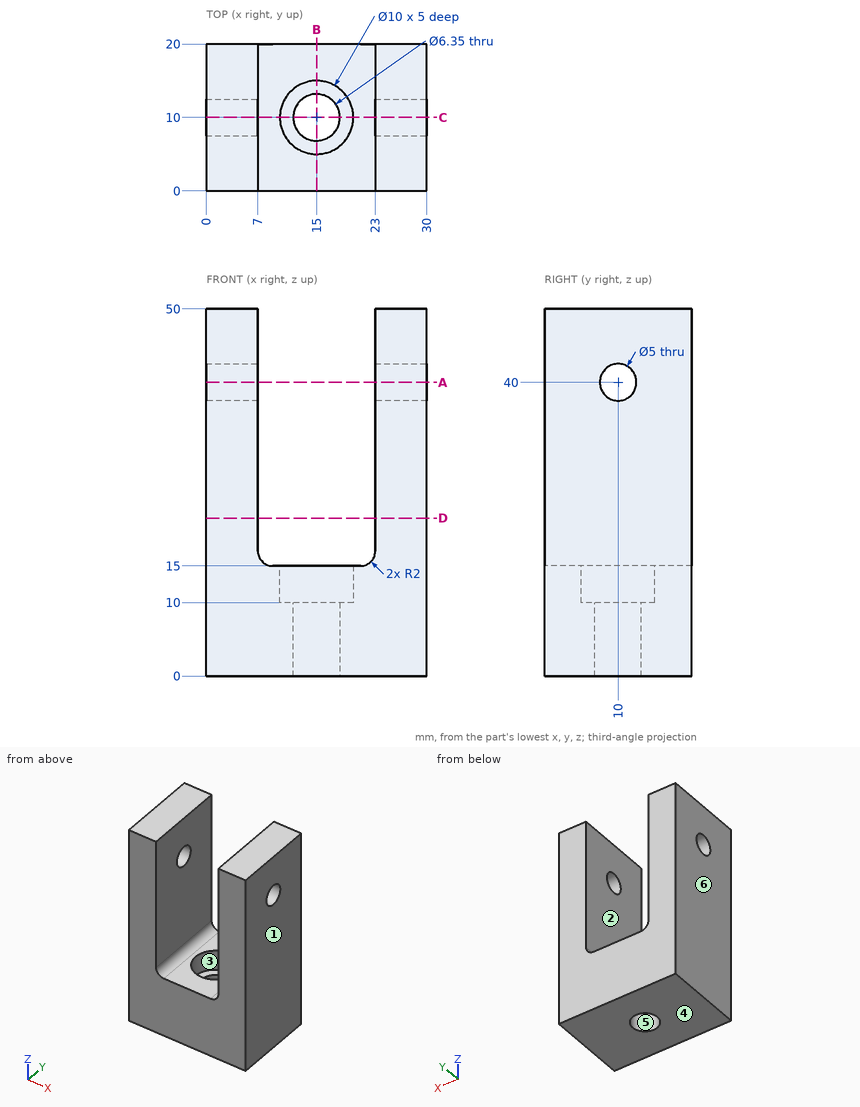
Geometry: see drawing. Coordinates: mm, zero at the bounding-box minimum. A direction names the side the tool comes from. Round coordinates to 2 decimals unless told otherwise and drop trailing zeros. Write each loop counter-clockwise with the first axis right and the second up, starting at its lowest first coordinate (ties: lowest second). Pieces come first, ordered by that corner, then holes.
Item 1: Section query A-A (z = 40). Return loops of the section in (x, y), plus the area to 3 significant figures.
Item 2: Section query B-B (x = 15). Return loops of the section in (y, z) (3 decimals).
Item 3: Section query C-C (y = 10). Return loops of the section in (x, z) (3 decimals), plus the area to 3 significant figures.
Item 4: Section query D-D (z = 21.5). Return loops of the section in (x, y).
Item 5: Pin query (flat end, axial travel): P1, Ø6.5, axis at y = 10, z = 40, coming from the +X side; P2, Ø8.5, axis at x = 15, y = 10, coming from the +Z side; P3, Ø6, axis at x = 18, y = 5, coming from the +Z side. Return the tip coordinate at first contact, or that it passes through.
Item 6: Material intervals for L1, parallel to Y at x = 15, z = 13.35; L2, parallel to X at y = 13.5, z = 39.5; L3, parallel to Y at x = 5, z = 40, sorted ascending.
Item 7: Set-up query: the marked faces 1, 2 and 3. Return all of +Z, -Z, +X, -X, +Y, -Y with unobstructed straight access to the full face (end or side cutting, diameter ignored); none if empty.
Item 8: Mould query, pull axis X, two halves, no side actions, for the marked faces 4, 5 and 6. Classes: +X half, -X half, draft (parallel to the pull), parting line (faces both ways), or undercut.
Completed:
1. outline: (0, 0) - (7, 0) - (7, 7.5) - (0, 7.5) - close; (0, 12.5) - (7, 12.5) - (7, 20) - (0, 20) - close; (23, 0) - (30, 0) - (30, 7.5) - (23, 7.5) - close; (23, 12.5) - (30, 12.5) - (30, 20) - (23, 20) - close
1. area: 210 mm2
2. outline: (0, 0) - (6.825, 0) - (6.825, 10) - (5, 10) - (5, 15) - (0, 15) - close; (13.175, 0) - (20, 0) - (20, 15) - (15, 15) - (15, 10) - (13.175, 10) - close
3. outline: (0, 0) - (11.825, 0) - (11.825, 10) - (10, 10) - (10, 15) - (9, 15) arc R2 cw to (7, 17) - (7, 37.5) - (0, 37.5) - close; (0, 42.5) - (7, 42.5) - (7, 50) - (0, 50) - close; (18.175, 0) - (30, 0) - (30, 37.5) - (23, 37.5) - (23, 17) arc R2 cw to (21, 15) - (20, 15) - (20, 10) - (18.175, 10) - close; (23, 42.5) - (30, 42.5) - (30, 50) - (23, 50) - close
3. area: 758 mm2
4. outline: (0, 0) - (7, 0) - (7, 20) - (0, 20) - close; (23, 0) - (30, 0) - (30, 20) - (23, 20) - close
5. P1: stops at x = 30
5. P2: stops at z = 10
5. P3: stops at z = 15
6. L1: y = 0 to 5, 15 to 20
6. L2: x = 0 to 7, 23 to 30
6. L3: y = 0 to 7.5, 12.5 to 20
7. face 1: +Z, -Z, +X, +Y, -Y
7. face 2: +Z, +Y, -Y
7. face 3: +Z
8. face 4: draft
8. face 5: undercut
8. face 6: -X half
